```python
from build123d import *

# Parameters (mm, degrees)
TORUS004_R        = 0.6
CYLINDER068_R     = 1.4
CYLINDER068_DEPTH = 2
ARRAY014_COUNT    = 3
CYLINDER067_R     = 13.5
CYLINDER067_DEPTH = 6
CYLINDER066_R     = 24
CYLINDER066_DEPTH = 2
CYLINDER065_R     = 17
CYLINDER065_DEPTH = 4


with BuildPart() as pot_rim_clip:
    # Torus004 → Torus004 (revolve)
    with BuildSketch(Plane(origin=(0, 0, 2.5), x_dir=(1, 0, 0), z_dir=(0, -1, 0))):
        with Locations((13.5, 0)):
            Circle(TORUS004_R)
    revolve(axis=Axis((0, 0, 2.5), (0, 0, 1)))


with BuildPart() as screw_holes001:
    # Cylinder068 → Cylinder068 (new body)
    with BuildSketch(Plane(origin=(20.5, 0, 0), x_dir=(1, 0, 0), z_dir=(0, 0, 1))):
        Circle(CYLINDER068_R)
    extrude(amount=CYLINDER068_DEPTH)

    # Array014: screw-holes001 ×3 about axis
    array014_axis = Axis((0, 0, 0), (0, 0, 1))


with BuildPart() as screw_holes001_1:
    add(screw_holes001.part)
    for i in range(1, ARRAY014_COUNT):
        add(screw_holes001.part.rotate(array014_axis, i * 360 / ARRAY014_COUNT))


with BuildPart() as pot_thread_hole001:
    # Cylinder067 → Cylinder067 (new body)
    with BuildSketch(Plane.XY):
        Circle(CYLINDER067_R)
    extrude(amount=CYLINDER067_DEPTH)


with BuildPart() as brim001:
    # Cylinder066 → Cylinder066 (new body)
    with BuildSketch(Plane.XY):
        Circle(CYLINDER066_R)
    extrude(amount=CYLINDER066_DEPTH)


with BuildPart() as pot_mount002:
    # Cylinder065 → Cylinder065 (new body)
    with BuildSketch(Plane.XY.offset(2)):
        Circle(CYLINDER065_R)
    extrude(amount=CYLINDER065_DEPTH)

    # Fusion028: union brim001
    add(brim001.part)

    # Cut049: cut pot-thread-hole001
    add(pot_thread_hole001.part, mode=Mode.SUBTRACT)

    # Cut053: cut screw-holes001
    add(screw_holes001_1.part, mode=Mode.SUBTRACT)

    # Fusion029: union pot-rim-clip
    add(pot_rim_clip.part)


with BuildPart() as pot_mount002_1:
    # Fusion029 placement: moved
    add(pot_mount002.part.moved(Location((0, 0, 30.2))))


solid = pot_mount002_1.part
```
The listing builds one solid part. Answer for the finished solid, in the listing's coordinates (mm). A direction names the side the tool comes from. Coordinates: 2 decimals unless noted, no trailing zeros. Write each loop counter-clockwise with the first axis right and the second up, starting at its lowest first coordinate (ties: lowest second). Pieces come first, ordered by that corner, then holes. Notation, with made-up numbers: (53, -26) - (90, -26) arc R21 cw to (90, 9) - close; hole circle Ø10 at (47, 40.5). An arc over 180 degrees is marked (long way). Return JSON: item names as keys, results as strings. Group by question number.
1. A cutting plane is placed at C-C, the plane x = 20.5. Determine the outline of the cut face in (y, z).
2. A cutting plane is placed at A-A, the plane y = 0. Determine the outline of the cut face in (x, z).
3. A cutting plane is placed at D-D, the plane x = -10.25. Give the number of separate pieces and of enclosed holes in the cut face, plus the area to 3 significant figures.
4. Which of the six approach directions +Z, -Z, +X, -X, +Y, -Y give full straight-line access (tool end or side, diameter ignored) to faces 5 (the cylindrical face through (-2.93, -13.18, 34.73)), 6 (the cylindrical face through (-11.361, -18.605, 31.186))?
5. Given pin 1 (1.5 mm diameter, centred on x = 9, z = 34.5, fed in from +Y); pin 2 (1 mm diameter, centred on x = 8.5, z = 31, fed in from -Y); pin 3 (1.5 mm diameter, centred on x = 9.5, z = 31, fed in from -Y), each flat-ended and moving along its own axis, determine where each tip first touches the part or whether it passes through.
6. A cutting plane is placed at B-B, the plane x = 0. Determine the outline of the cut face in (y, z), plus the area to 3 significant figures.
7. Determine the mould class of faces 1 (the flat face through (10, -10, 30.2)), 2 (the cylindrical face through (-2.93, -13.18, 31.14)), 3 (the cylindrical face through (9.139, 14.334, 34.172)), 4 (the cylindrical face through (-10.43, 19.14, 31.19)) for opening direction Y: released by +Y, released by -Y, zero draft, split by the parting line, or undercut.
8. Straight lines are drawn through the part: L1, parallel to Y at x = -10.25, z = 31.1; L2, parallel to Y at x = 0, z = 31.2; L3, parallel to Y at x = -12, z = 30.5. For each, find the intervals that lie inside material, in ascending order.
Ans:
{
 "1": {"outline": "(-12.48, 30.2) - (-1.4, 30.2) - (-1.4, 32.2) - (-12.48, 32.2) - close; (1.4, 30.2) - (12.48, 30.2) - (12.48, 32.2) - (1.4, 32.2) - close"},
 "2": {"outline": "(-24, 30.2) - (-13.5, 30.2) - (-13.5, 32.1) arc R0.6 ccw to (-13.5, 33.3) - (-13.5, 36.2) - (-17, 36.2) - (-17, 32.2) - (-24, 32.2) - close; (13.5, 30.2) - (19.1, 30.2) - (19.1, 32.2) - (17, 32.2) - (17, 36.2) - (13.5, 36.2) - (13.5, 33.3) arc R0.6 ccw to (13.5, 32.1) - close; (21.9, 30.2) - (24, 30.2) - (24, 32.2) - (21.9, 32.2) - close"},
 "3": {"separate pieces": "4", "enclosed holes": "0", "area": "80.5 mm²"},
 "4": {"face 5": "+Z", "face 6": "+Z, -Z"},
 "5": {"pin 1": "y = 14.86", "pin 2": "y = -22.63", "pin 3": "y = -22.35"},
 "6": {"outline": "(-24, 30.2) - (-13.5, 30.2) - (-13.5, 32.1) arc R0.6 ccw to (-13.5, 33.3) - (-13.5, 36.2) - (-17, 36.2) - (-17, 32.2) - (-24, 32.2) - close; (13.5, 30.2) - (24, 30.2) - (24, 32.2) - (17, 32.2) - (17, 36.2) - (13.5, 36.2) - (13.5, 33.3) arc R0.6 ccw to (13.5, 32.1) - close", "area": "71.1 mm²"},
 "7": {"face 1": "zero draft", "face 2": "undercut", "face 3": "split by the parting line", "face 4": "undercut"},
 "8": {"L1": "-21.7 to -19.15, -16.35 to -8.79, 8.79 to 16.35, 19.15 to 21.7", "L2": "-24 to -13.5, 13.5 to 24", "L3": "-20.78 to -6.18, 6.18 to 20.78"}
}
